Model file for the job. Use its own axes, mm. A direction names the side the tool comes from. Coordinates: 2 decimals unless noted, no trailing zeros. Order: outer loops, then holes, each group sorted by start corner. A loop starts at its lowest first (then second) coordinate and runs counter-clockwise, first axis right, second up. Notation, with made-up numbers: M 53.5,-8 L 60.5,-8 A14 cw 60.5,-4 Z; hole C -1.75,44 d11. An arc over 180 degrees is marked long. Return JSON: item names as keys, results as strings.
```python
from build123d import *

# Parameters (mm, degrees)
SKETCH1_R           = 3.75
SKETCH1_W           = 89.5
SKETCH1_H           = 42
BOSS_EXTRUDE1_DEPTH = 3.2
CHAMFER1_SIZE       = 2.4
CHAMFER1_SIZE2      = 0.99411255
SKETCH3_W           = 15
SKETCH3_H           = 15
CUT_EXTRUDE2_DEPTH  = 0.8
SKETCH4_R           = 6.5
CUT_EXTRUDE3_DEPTH  = 0.9


with BuildPart() as part:
    # Sketch1 → Boss-Extrude1 (new body)
    with BuildSketch(Plane.XY):
        Polygon((-9.75, 56.5), (99.25, 56.5), (119.25, 56.5), (119.25, -14.5), (99.25, -14.5), (-9.75, -14.5), align=None)
        with Locations((104.25, 21)):
            Circle(SKETCH1_R, mode=Mode.SUBTRACT)
        with Locations((44.75, 21)):
            Rectangle(SKETCH1_W, SKETCH1_H, mode=Mode.SUBTRACT)
    extrude(amount=BOSS_EXTRUDE1_DEPTH)

    # Chamfer1
    chamfer1_edges = [part.edges().sort_by_distance(p)[0] for p in [
        (54.75, 56.5, 3.2),
    ]]
    chamfer1_side = [part.faces().sort_by_distance(p)[0] for p in [
        (54.75, 56.5, 1.6),
    ]]
    chamfer(chamfer1_edges, length=CHAMFER1_SIZE, length2=CHAMFER1_SIZE2, reference=chamfer1_side[0])

    # Sketch3 → Cut-Extrude2 (cut)
    with BuildSketch(Plane(origin=(0, 0, 0), x_dir=(-1, 0, 0), z_dir=(0, 0, -1))):
        with Locations((-104.25, 21)):
            Rectangle(SKETCH3_W, SKETCH3_H)
    extrude(amount=-CUT_EXTRUDE2_DEPTH, mode=Mode.SUBTRACT)

    # Sketch4 → Cut-Extrude3 (cut)
    with BuildSketch(Plane.XY.offset(3.2)):
        with Locations((104.25, 21)):
            Circle(SKETCH4_R)
    extrude(amount=-CUT_EXTRUDE3_DEPTH, mode=Mode.SUBTRACT)


solid = part.part
```
Item 1: Saw through at B-B (x = 104.25). Write the cut outline in (y, z), and give its area (3 significant figures).
Check result:
{"outline": "M -14.5,0 L 13.5,0 L 13.5,0.8 L 17.25,0.8 L 17.25,2.3 L 14.5,2.3 L 14.5,3.2 L -14.5,3.2 Z; M 24.75,0.8 L 28.5,0.8 L 28.5,0 L 56.5,0 L 56.5,0.8 L 55.51,3.2 L 27.5,3.2 L 27.5,2.3 L 24.75,2.3 Z", "area": "191 mm2"}
Item 2: 3-axis set-ups, long thin cutter, end or side, ignore diameter. For faces 4 (the flat face through (44, 42, 2)), 5 (the flat face through (119.25, 21, 2)), 6 (the flat face through (107, 18, 2.3)), 7 (the flat face through (108, 23, 0.8)): which of +Z, -Z, +X, -X, +Y, -Y reach the whole face in a straight line?
Check result:
{"face 4": "+Z, -Z", "face 5": "+Z, -Z, +X, +Y, -Y", "face 6": "+Z", "face 7": "-Z"}
Item 3: Pull direction Y, two halves, no side cores. Call faces 1 (the flat face through (54, -14.5, 2)), 2 (the flat face through (-9.75, 21, 2)), 3 (the cylindrical face through (110.45, 22.95, 2.76)): +Y half, -Y half, draft (parallel to the pull), parting line (faces both ways), or undercut.
Check result:
{"face 1": "-Y half", "face 2": "draft", "face 3": "undercut"}
Item 4: Saw through at D-D (z = 1.35). Write the cut outline in (x, y), and give its area (3 significant figures).
Check result:
{"outline": "M -9.75,-14.5 L 119.25,-14.5 L 119.25,56.27 L -9.75,56.27 Z; hole M 0,0 L 89.5,0 L 89.5,42 L 0,42 Z; hole C 104.25,21 d7.5", "area": "5,330 mm2"}
Item 5: Saw through at A-A (y = 8). Write the cut outline in (x, z), and give its area (3 significant figures).
Check result:
{"outline": "M -9.75,0 L 0,0 L 0,3.2 L -9.75,3.2 Z; M 89.5,0 L 119.25,0 L 119.25,3.2 L 89.5,3.2 Z", "area": "126 mm2"}
Item 6: Drop flat-ended pins along their axis: pin 1 Ø16.5 at (x, y) = (103.5, 23) entering from -Z; pin 2 Ø1 at (x, z) = (23, 2) entering from +Y; pin 3 Ø6 at (x, y) = (104.25, 21) entering from -Z (3 decimals). Give the stop position or say it passes through.
Check result:
{"pin 1": "stops at z = 0", "pin 2": "stops at y = 56.21", "pin 3": "passes through"}
Item 7: Saw through at C-C (y = 21). Write the cut outline in (x, z).
Check result:
{"outline": "M -9.75,0 L 0,0 L 0,3.2 L -9.75,3.2 Z; M 89.5,0 L 96.75,0 L 96.75,0.8 L 100.5,0.8 L 100.5,2.3 L 97.75,2.3 L 97.75,3.2 L 89.5,3.2 Z; M 108,0.8 L 111.75,0.8 L 111.75,0 L 119.25,0 L 119.25,3.2 L 110.75,3.2 L 110.75,2.3 L 108,2.3 Z"}
Item 8: Wall check: line 1 (X direction, y = 21, z = 0.75); line 2 (X direction, y = 13, z = 2.4); line 3 (X direction, y = 21, z = 1.35). Give the ranges that are in metal, low to high.
Check result:
{"line 1": "x = -9.75 to 0, 89.5 to 96.75, 111.75 to 119.25", "line 2": "x = -9.75 to 0, 89.5 to 119.25", "line 3": "x = -9.75 to 0, 89.5 to 100.5, 108 to 119.25"}
